Verification items for the finished model (mm, model axes). A direction names the side the tool comes from. Round coordinates to 2 decimals unless told otherwise and drop trailing zeros. Order: outer loops, then holes, each group sorted by start corner. A loop starts at its lowest first (then second) coordinate and runs counter-clockwise, first axis right, second up. Notation, with made-up numbers: M 58.25,6 L 64.25,6 A24 ccw 64.25,28 Z; hole C 80,9.25 d10. An arc over 180 degrees is marked long. Use CSV: the item, a comma, the result in double quotes. Start each with the question number.
Q1. Gauge pin test, flat ends, axial feed: pin 1 Ø6 at (x, y) = (21, -4) entering from +Z; pin 2 Ø12 at (x, z) = (10.5, 15) entering from -Y. Record the tip position at first contact, or that the pin passes through.
Q2. Sectioned sample at D-D (y = -4). Enter the section's corners in (x, z).
Q3. Scan lines: line 1 (Y direction, x = 47.2, z = 13); line 2 (X direction, y = -10.25, z = 6); line 3 (Z direction, x = 41, y = -12.75). Record each from-to range of solid material in increasing order.
Q4. Sectioned sample at C-C (z = 13). Enter the section's corners in (x, y).
Q5. Sectioned sample at A-A (y = -10). Enter the section's corners in (x, z), and give its area (3 significant figures).
Q6. Sectioned sample at B-B (z = 17.5). Enter the section's corners in (x, y).
Q7. Mould release check, pull along Y, two halves, no side actions. Record for faces 1 (the face through (24, -10, 0)), 2 (the face through (47.27, -11.05, 10.46)), 3 (the face through (24, -20, 4)): +Y half, -Y half, draft (parallel to the pull), parting line (faces both ways), or undercut.
Q8. Set-up check for faces 4 (the face through (4, -10, 15)), 5 (the face through (48, -10, 25)): record each of +Z, -Z, +X, -X, +Y, -Y from which the full face is reachable in a straight line by a thin tool's end or side.
```python
from build123d import *

# Parameters (mm, degrees)
SKETCH_1_W          = 49.5
SKETCH_1_H          = 20
EXTRUDE_1_DEPTH     = 5
SKETCH_3_W          = 4
SKETCH_3_H          = 20
EXTRUDE_2_DEPTH     = 20
CHAMFER_1_SIZE      = 0.5
SKETCH_4_R          = 2.75
CUT_EXTRUDE_1_DEPTH = 20
CHAMFER_2_SIZE      = 0.5


with BuildPart() as part:
    # 草图1 → 凸台-拉伸1 (new body)
    with BuildSketch(Plane.XY):
        with Locations((24.75, -10)):
            Rectangle(SKETCH_1_W, SKETCH_1_H)
    extrude(amount=EXTRUDE_1_DEPTH)

    # 草图3 → 凸台-拉伸2 (add)
    with BuildSketch(Plane.XY.offset(5)):
        with Locations((47.5, -10)):
            Rectangle(SKETCH_3_W, SKETCH_3_H)
        with Locations((2, -10)):
            Rectangle(SKETCH_3_W, SKETCH_3_H)
    extrude(amount=EXTRUDE_2_DEPTH)

    # 倒角1
    chamfer_1_edges = [part.edges().sort_by_distance(p)[0] for p in [
        (45.5, -10, 25),
        (4, -10, 25),
    ]]
    chamfer(chamfer_1_edges, length=CHAMFER_1_SIZE)

    # 草图4 → 切除-拉伸1 (cut)
    with BuildSketch(Plane(origin=(49.5, 0, 0), x_dir=(0, 0, -1), z_dir=(1, 0, 0))):
        with Locations((-13, -10)):
            Circle(SKETCH_4_R)
    extrude(amount=-CUT_EXTRUDE_1_DEPTH, mode=Mode.SUBTRACT)

    # 倒角2
    chamfer_2_edges = [part.edges().sort_by_distance(p)[0] for p in [
        (49.5, -10, 15.75),
    ]]
    chamfer(chamfer_2_edges, length=CHAMFER_2_SIZE)


solid = part.part
```
Verdict:
1,pin 1,"stops at z = 5"
1,pin 2,"passes through"
2,outline,"M 0,0 L 49.5,0 L 49.5,25 L 46,25 L 45.5,24.5 L 45.5,5 L 4,5 L 4,24.5 L 3.5,25 L 0,25 Z"
3,line 1,"y = -20 to -12.75, -7.25 to 0"
3,line 2,"x = 0 to 4, 45.5 to 49.5"
3,line 3,"z = 0 to 5"
4,outline,"M 0,-20 L 4,-20 L 4,0 L 0,0 Z; M 45.5,-20 L 49.5,-20 L 49.5,-13.25 L 49,-12.75 L 45.5,-12.75 Z; M 45.5,-7.25 L 49,-7.25 L 49.5,-6.75 L 49.5,0 L 45.5,0 Z"
5,outline,"M 0,0 L 49.5,0 L 49.5,9.75 L 49,10.25 L 45.5,10.25 L 45.5,5 L 4,5 L 4,24.5 L 3.5,25 L 0,25 Z; M 45.5,15.75 L 49,15.75 L 49.5,16.25 L 49.5,25 L 46,25 L 45.5,24.5 Z"
5,area,"385 mm²"
6,outline,"M 0,-20 L 4,-20 L 4,0 L 0,0 Z; M 45.5,-20 L 49.5,-20 L 49.5,0 L 45.5,0 Z"
7,face 1,"draft"
7,face 2,"undercut"
7,face 3,"-Y half"
8,face 4,"+Z, +Y, -Y"
8,face 5,"+Z, +X, -X, +Y, -Y"
